Design review of the part built by this model. Coordinates are the model's own, in mm. A direction names the side the tool comes from. Coordinates: 2 decimals unless noted, no trailing zeros. Loops run counter-clockwise (first coordinate to the right, second up) from the corner with the lowest first, then second, coordinate; pieces in that order, holes last. Notation, with made-up numbers: M 21,78 L 41,78 A7 cw 41,87 Z; hole C 13.5,-5.75 d6. An arc over 180 degrees is marked long. Put each result on its own line as item: value. Start each with the question number.
(1) For probe 1 along Z at (x, y) = (1.2, 152); probe 2 along Y at (x, z) = (3, 201); probe 3 along Y at (x, z) = (0.4, 188.5), list the stretches that pass through material, from the lowest coordinate up. Write a range as [from, to].
(2) The part is to be moulded in two halves that separate along Y. For faces 3 (the cylindrical face through (2.13, 225.7, 294.62)), 4 (the cylindrical face through (2.13, 147.4, 267.12)), 5 (the flat face through (4.318, 115, 203)), 6 (the flat face through (2.13, 76.9, 113.43)), say which applies: +Y half, -Y half, draft (parallel to the pull), parting line (faces both ways), or undercut.
(3) Take a section at B-B, the plane z = 210. Give the boundary of the cut face in (x, y).
(4) Take a section at A-A, the plane x = 2.9. Count the separate pieces of the cut face and the enclosed holes in it, then the cut area to 3 significant figures.
(5) For faces 1 (the flat face through (2.13, 40.09, 264.4)), 2 (the flat face through (2.129, 1.868, 181.766)), list the 3-axis set-ups (+Z, -Z, +X, -X, +Y, -Y) from which the entire face can be reached by the end or side of a thin tool; tool diameter is ignored.
(6) Clearance check with flat-ended pins moving along their axes: pin 1 (5 mm diameter, centred on y = 162.43, z = 286.37, fed in from +X); pin 2 (2 mm diameter, centred on x = 1.5, z = 167, fed in from +Y); pin 3 (2 mm diameter, centred on x = 1.5, z = 186, fed in from -Y). State where each tip first meets the part, or that it passes through.
```python
from build123d import *

# Parameters (mm, degrees)
SKETCH2_R           = 2.38125
SKETCH2_R_2         = 1.850000002
SKETCH2_R_3         = 1.85
SKETCH2_R_4         = 1.778
SKETCH2_R_5         = 1.8415
BOSS_EXTRUDE1_DEPTH = 4.318


with BuildPart() as part:
    # Sketch2 → Boss-Extrude1 (new body)
    with BuildSketch(Plane(origin=(0, 0, 0), x_dir=(0, 0, -1), z_dir=(1, 0, 0))):
        with BuildLine():
            Line((-115.889220019, 171.954), (-189.580583869, 171.954))
            Line((-189.580583869, 171.954), (-230.07024685, 220.207701322))
            ThreePointArc((-230.07024685, 220.207701322), (-232.251003102, 221.881054448), (-234.934629064, 222.476))
            Line((-234.934629064, 222.476), (-250.119258716, 222.476))
            Line((-250.119258716, 222.476), (-259.069094553, 226.862369804))
            ThreePointArc((-259.069094553, 226.862369804), (-260.42931468, 227.346249494), (-261.863679558, 227.510370624))
            Line((-261.863679558, 227.510370624), (-290.181258716, 227.510370624))
            ThreePointArc((-290.181258716, 227.510370624), (-294.671386777, 225.650498684), (-296.531258716, 221.160370624))
            Line((-296.531258716, 221.160370624), (-296.531258716, 57.430370624))
            ThreePointArc((-296.531258716, 57.430370624), (-294.538216111, 51.386662581), (-289.341021135, 47.714089896))
            Line((-289.341021135, 47.714089896), (-238.759677477, 32.254))
            Line((-238.759677477, 32.254), (-202.359677477, -1.524))
            Line((-202.359677477, -1.524), (-189.491289728, -1.524))
            Line((-189.491289728, -1.524), (-183.278653236, 7.686612375))
            Line((-183.278653236, 7.686612375), (-179.541351859, 5.165770766))
            Line((-179.541351859, 5.165770766), (-184.053659217, -1.524))
            Line((-184.053659217, -1.524), (-158.188157254, -1.524))
            ThreePointArc((-158.188157254, -1.524), (-155.726821474, -1.027573796), (-153.650327137, 0.384086243))
            Line((-153.650327137, 0.384086243), (-122.571428599, 32.134086243))
            ThreePointArc((-122.571428599, 32.134086243), (-121.22972977, 34.177325496), (-120.759258716, 36.576))
            Line((-120.759258716, 36.576), (-120.759258716, 66.032))
            Line((-120.759258716, 66.032), (-105.889220019, 88.077738973))
            Line((-105.889220019, 88.077738973), (-105.889220019, 161.954))
            ThreePointArc((-105.889220019, 161.954), (-108.818152207, 169.025067812), (-115.889220019, 171.954))
        make_face()
        with Locations((-243.629318942, 168.931188955)):
            Circle(SKETCH2_R, mode=Mode.SUBTRACT)
        with Locations((-286.371258716, 57.430370624)):
            Circle(SKETCH2_R, mode=Mode.SUBTRACT)
        with Locations((-229.557259723, 141.660587995)):
            Circle(SKETCH2_R, mode=Mode.SUBTRACT)
        with Locations((-112.732319415, 86.216867446)):
            Circle(SKETCH2_R_2, mode=Mode.SUBTRACT)
        with Locations((-199.955990958, 72)):
            Circle(SKETCH2_R_3, mode=Mode.SUBTRACT)
        with Locations((-199.955990958, 152)):
            Circle(SKETCH2_R_3, mode=Mode.SUBTRACT)
        with Locations((-199.955990958, 168)):
            Circle(SKETCH2_R_3, mode=Mode.SUBTRACT)
        with Locations((-221.371258716, 36.430370624)):
            Circle(SKETCH2_R_4, mode=Mode.SUBTRACT)
        with Locations((-240.13308557, 87.518200818)):
            Circle(SKETCH2_R, mode=Mode.SUBTRACT)
        with Locations((-199.955990958, 40)):
            Circle(SKETCH2_R_3, mode=Mode.SUBTRACT)
        with Locations((-191.955990958, 48)):
            Circle(SKETCH2_R_3, mode=Mode.SUBTRACT)
        with Locations((-199.955990958, 56)):
            Circle(SKETCH2_R_3, mode=Mode.SUBTRACT)
        with Locations((-280.371258716, 125.430370624)):
            Circle(SKETCH2_R_5, mode=Mode.SUBTRACT)
        with Locations((-222.371258716, 159.430370624)):
            Circle(SKETCH2_R_5, mode=Mode.SUBTRACT)
        with Locations((-286.371258716, 162.430370624)):
            Circle(SKETCH2_R_5, mode=Mode.SUBTRACT)
        with Locations((-265.366688027, 145.789251152)):
            Circle(SKETCH2_R, mode=Mode.SUBTRACT)
        with Locations((-234.371258716, 217.430370624)):
            Circle(SKETCH2_R_5, mode=Mode.SUBTRACT)
        with Locations((-290.871258716, 222.430370624)):
            Circle(SKETCH2_R_5, mode=Mode.SUBTRACT)
        with BuildLine():
            Line((-287.829388906, 193.285058383), (-284.701870397, 193.761043975))
            ThreePointArc((-284.701870397, 193.761043975), (-282.046244193, 195.026852777), (-280.537562028, 197.552422136))
            ThreePointArc((-280.537562028, 197.552422136), (-272.673389463, 208.141620232), (-259.619652409, 210.032724503))
            ThreePointArc((-259.619652409, 210.032724503), (-258.077063161, 209.822786209), (-256.52721589, 209.969854606))
            ThreePointArc((-256.52721589, 209.969854606), (-253.968498332, 209.529478199), (-252.417164512, 207.447572749))
            ThreePointArc((-252.417164512, 207.447572749), (-251.846450969, 205.99914542), (-250.960720569, 204.718857431))
            ThreePointArc((-250.960720569, 204.718857431), (-253.704909037, 179.546702846), (-278.544971255, 184.459873489))
            ThreePointArc((-278.544971255, 184.459873489), (-280.736689043, 186.422268863), (-283.64864912, 186.840731487))
            Line((-283.64864912, 186.840731487), (-286.776167629, 186.364745894))
            ThreePointArc((-286.776167629, 186.364745894), (-290.762934512, 189.2982915), (-287.829388906, 193.285058383))
        make_face(mode=Mode.SUBTRACT)
        with BuildLine():
            Line((-177.859990958, 39.62), (-191.067990958, 39.62))
            ThreePointArc((-191.067990958, 39.62), (-192.504831938, 39.024840979), (-193.099990958, 37.588))
            Line((-193.099990958, 37.588), (-193.099990958, 24.158))
            ThreePointArc((-193.099990958, 24.158), (-192.504831938, 22.721159021), (-191.067990958, 22.126))
            Line((-191.067990958, 22.126), (-177.859990958, 22.126))
            ThreePointArc((-177.859990958, 22.126), (-176.423149979, 22.721159021), (-175.827990958, 24.158))
            Line((-175.827990958, 24.158), (-175.827990958, 37.588))
            ThreePointArc((-175.827990958, 37.588), (-176.423149979, 39.024840979), (-177.859990958, 39.62))
        make_face(mode=Mode.SUBTRACT)
    extrude(amount=BOSS_EXTRUDE1_DEPTH)


solid = part.part
```
Computed values:
1. probe 1: z = [105.89, 198.11], [201.81, 296.53]
1. probe 2: y = [-1.52, 38.47], [41.53, 54.47], [57.53, 70.47], [73.53, 150.47], [153.53, 166.47], [169.53, 185.56]
1. probe 3: y = [-0.05, 22.13], [39.62, 171.95]
2. face 3: +Y half
2. face 4: undercut
2. face 5: draft
2. face 6: -Y half
3. outline: M 0,5.57 L 4.32,5.57 L 4.32,196.29 L 0,196.29 Z
4. separate pieces: 1
4. enclosed holes: 20
4. area: 31,100 mm^2
5. face 1: +Z, +X, -X, -Y
5. face 2: +X, -X
6. pin 1: stops at x = 4.32
6. pin 2: stops at y = 171.95
6. pin 3: stops at y = 2.17
